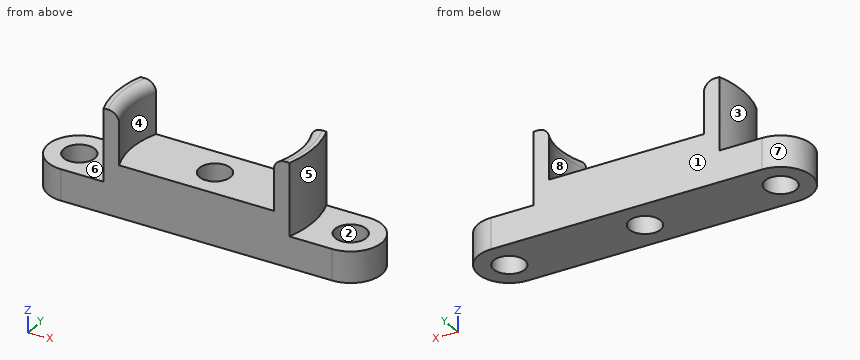
from build123d import *

# Parameters (mm, degrees)
SKETCH_2_W          = 49.66242786768973
SKETCH_2_H          = 43.948008528228435
CUT_EXTRUDE_1_DEPTH = 10
SKETCH_3_R          = 1.5
SKETCH_3_R_2        = 1.5000000000000007
SKETCH_3_R_3        = 1.5000000000000004
CUT_EXTRUDE_2_DEPTH = 18.029386365926428
EXTRUDE_START       = 5
EXTRUDE_2_DEPTH     = 5
FILLET_2_R          = 1


with BuildPart() as part:
    # 草图1 → 旋转3 (revolve)
    with BuildSketch(Plane(origin=(0, 0, 0), x_dir=(1, 0, 0), z_dir=(0, 1, 0)), mode=Mode.PRIVATE) as revolve_3_sk:
        Polygon((0, 0), (0, 5.000000000000001), (20, 5.000000000000001), (20, 2.0000000000000018), (9.4, 2.0000000000000004), (9.4, 2.6e-16), align=None)
    revolve(revolve_3_sk.sketch.rotate(Axis((0, 0, 0), (0, 0, 1)), 180), axis=Axis((0, 0, 0), (0, 0, 1)))

    # 草图2 → 切除-拉伸1 (cut)
    with BuildSketch(Plane.XY):
        Rectangle(SKETCH_2_W, SKETCH_2_H)
        with BuildLine():
            Line((13, -2.999999999999997), (-13, -3))
            ThreePointArc((-13, -3), (-16, 3.7e-16), (-13, 3))
            Line((-13, 3), (13, 3.000000000000003))
            ThreePointArc((13, 3.000000000000003), (16, 3.18e-15), (13, -2.999999999999997))
        make_face(mode=Mode.SUBTRACT)
    extrude(amount=-CUT_EXTRUDE_1_DEPTH, mode=Mode.SUBTRACT)

    # 草图3 → 切除-拉伸2 (cut, through all)
    with BuildSketch(Plane.XY):
        Circle(SKETCH_3_R)
        with Locations((12.999999999999998, 0)):
            Circle(SKETCH_3_R_2)
        with Locations((-13.000000000000002, 0)):
            Circle(SKETCH_3_R_3)
    extrude(amount=-CUT_EXTRUDE_2_DEPTH, mode=Mode.SUBTRACT)

    # 草图5 → 凸台-拉伸2 (add)
    with BuildSketch(Plane.XY.offset(EXTRUDE_START)):
        with BuildLine():
            Line((-7.416198487095722, 3.0000000000000004), (-8.908422980528035, 3.0000000000000004))
            ThreePointArc((-8.908422980528037, 3.000000000000001), (-9.400000000000002, 5.6e-16), (-8.90842298052804, -3))
            Line((-8.908422980528037, -2.9999999999999996), (-7.416198487095721, -2.9999999999999996))
            ThreePointArc((-7.416198487095696, -2.9999999999999187), (-8, 9.8e-16), (-7.416198487095695, 2.9999999999999205))
        make_face()
        with BuildLine():
            Line((8.908422980528035, 3.000000000000002), (7.41619848709553, 3.000000000000002))
            ThreePointArc((7.416198487095587, 3.000000000000189), (7.852693419991789, 1.5281380996551506), (8, 0))
            ThreePointArc((8, -1.96e-15), (7.85269341999179, -1.5281380996551457), (7.416198487095591, -3.0000000000001785))
            Line((7.416198487095535, -2.999999999999998), (8.908422980528037, -2.999999999999998))
            ThreePointArc((8.908422980528037, -2.999999999999998), (9.400000000000002, 1.67e-15), (8.908422980528037, 3.0000000000000018))
        make_face()
    extrude(amount=-EXTRUDE_2_DEPTH)

    # 圆角2
    fillet_2_edges = [part.edges().sort_by_distance(p)[0] for p in [
        (-8.000000000000002, 1.22e-15, 5),
        (8, 6.72e-15, 5),
    ]]
    fillet(fillet_2_edges, radius=FILLET_2_R)


solid = part.part
Can you work these out from the model? Positions are in its coordinate system, mm. Face numbers are marked on the shaded views. A direction names the side the tool comes from. Give positions to 0.01 mm unless a question says otherwise; leave off trailing zeros. Order: outer loops, then holes, each group sorted by start corner. A loop starts at its lowest first (then second) coordinate and runs counter-clockwise, first axis right, second up. Notation, with made-up numbers: M -24,88 L 29,88 A16 ccw 29,103 Z; hole C 8.5,79 d8. An arc over 180 degrees is marked long. Use a Markdown table: item, result. Add a question column.
Item 1: Suppose I cut it at A-A (z = 2.75). List the corners of the cut face in (x, y) for me.
Item 2: Suppose I cut it at B-B (y = 0). List the corners of the cut face in (x, z) for me.
Item 3: For the marked faces 1, 2, 3, 4 and 5, which set-ups out of +Z, -Z, +X, -X, +Y, -Y let a thin tool reach every point of the face, with its end or its side?
Item 4: We'd pull the mould along X, two halves only. Please class the marked faces 6, 7 and 8: +X half, -X half, draft (parallel to the pull), parting line (faces both ways), or undercut.
Item 5: If I drill on L1, parallel to Y at x = 0, z = -2.15; L2, parallel to X at y = -1.25, z = -3; L3, parallel to Z at x = -3, y = -0.5, over which ranges is the centre line in solid material (lowest first)? Write a range as [from, to].
Item 6: Suppose I cut it at C-C (x = 0). List the corners of the cut face in (y, z) for me.
Item 7: Suppose I cut it at D-D (z = -0.75). List the corners of the cut face in (x, y) for me.
Item 8: Will these pins go through, and if not, where does the flat tip stop? pin 1 (1.5 mm diameter, centred on x = 3, y = -0.5, fed in from +Z); pin 2 (2 mm diameter, centred on y = -1.5, z = -0.5, fed in from -X).
Answer sheet:
| question | item | result |
|---|---|---|
| 1 | outline | M -8.91,-3 L -7.42,-3 A8 cw -7.42,3 L -8.91,3 A9.4 ccw Z; M 7.42,-3 L 8.91,-3 A9.4 ccw 8.91,3 L 7.42,3 A8 cw Z |
| 2 | outline | M -16,-5 L -14.5,-5 L -14.5,-2 L -16,-2 Z; M -11.5,-5 L -1.5,-5 L -1.5,0 L -8,0 L -8,4 A1 ccw -9,5 L -9.4,5 L -9.4,-2 L -11.5,-2 Z; M 1.5,-5 L 11.5,-5 L 11.5,-2 L 9.4,-2 L 9.4,5 L 9,5 A1 ccw 8,4 L 8,0 L 1.5,0 Z; M 14.5,-5 L 16,-5 L 16,-2 L 14.5,-2 Z |
| 3 | face 1 | +Z, -Z, +X, -X, +Y |
| 3 | face 2 | +Z, -Z |
| 3 | face 3 | +Z, -X |
| 3 | face 4 | +Z |
| 3 | face 5 | +Z, +X |
| 4 | face 6 | draft |
| 4 | face 7 | -X half |
| 4 | face 8 | undercut |
| 5 | L1 | y = [-3, -1.5], [1.5, 3] |
| 5 | L2 | x = [-15.73, -13.83], [-12.17, -0.83], [0.83, 12.17], [13.83, 15.73] |
| 5 | L3 | z = [-5, 0] |
| 6 | outline | M -3,-5 L -1.5,-5 L -1.5,0 L -3,0 Z; M 1.5,-5 L 3,-5 L 3,0 L 1.5,0 Z |
| 7 | outline | M -8.91,-3 L 8.91,-3 A9.4 ccw 8.91,3 L -8.91,3 A9.4 ccw Z; hole C 0,0 d3 |
| 8 | pin 1 | stops at z = 0 |
| 8 | pin 2 | stops at x = -9.39 |
